```python
from build123d import *

# Parameters (mm, degrees)
F0_W     = 31.75
F0_H     = 57.15
F1_DEPTH = 50.8
F2_W     = 31.75
F2_H     = 25.4
F2_H_2   = 63.5
F3_DEPTH = 38.1
F4_W     = 63.5
F4_H     = 63.5
F5_DEPTH = 12.7
F7_DEPTH = 12.7


with BuildPart() as f1:
    # F0 (on Front) → F1 (new body)
    with BuildSketch(Plane.XZ):
        with BuildLine():
            Line((-13.088717841, 62.5215394646), (-70.238717841, 62.5215394646))
            Line((-70.238717841, 62.5215394646), (-70.238717841, 25.6915394646))
            ThreePointArc((-70.238717841, 25.6915394646), (-55.8703080473, 19.7399492583), (-49.918717841, 5.3715394646))
            Line((-49.918717841, 5.3715394646), (-13.088717841, 5.3715394646))
            Line((-13.088717841, 5.3715394646), (-13.088717841, 62.5215394646))
        make_face()
        with BuildLine():
            Line((-13.088717841, -51.7784605354), (-13.088717841, 5.3715394646))
            Line((-13.088717841, 5.3715394646), (-49.918717841, 5.3715394646))
            ThreePointArc((-49.918717841, 5.3715394646), (-55.8703080473, -8.9968703291), (-70.238717841, -14.9484605354))
            Line((-70.238717841, -14.9484605354), (-70.238717841, -51.7784605354))
            Line((-70.238717841, -51.7784605354), (-13.088717841, -51.7784605354))
        make_face()
        with BuildLine():
            Line((87.241282159, 5.3715394646), (50.411282159, 5.3715394646))
            Line((50.411282159, 5.3715394646), (50.411282159, -51.7784605354))
            Line((50.411282159, -51.7784605354), (107.561282159, -51.7784605354))
            Line((107.561282159, -51.7784605354), (107.561282159, -14.9484605354))
            ThreePointArc((107.561282159, -14.9484605354), (93.1928723653, -8.9968703291), (87.241282159, 5.3715394646))
        make_face()
        with BuildLine():
            Line((107.561282159, 62.5215394646), (50.411282159, 62.5215394646))
            Line((50.411282159, 62.5215394646), (50.411282159, 5.3715394646))
            Line((50.411282159, 5.3715394646), (87.241282159, 5.3715394646))
            ThreePointArc((87.241282159, 5.3715394646), (93.1928723653, 19.7399492583), (107.561282159, 25.6915394646))
            Line((107.561282159, 25.6915394646), (107.561282159, 62.5215394646))
        make_face()
        with Locations((2.786282159, 33.9465394646)):
            Rectangle(F0_W, F0_H)
        with Locations((2.786282159, -23.2034605354)):
            Rectangle(F0_W, F0_H)
        with Locations((34.536282159, -23.2034605354)):
            Rectangle(F0_W, F0_H)
        with Locations((34.536282159, 33.9465394646)):
            Rectangle(F0_W, F0_H)
    extrude(amount=-F1_DEPTH)

    # F2 (on face) → F3 (join)
    with BuildSketch(Plane.XZ):
        with Locations((34.536282159, 49.8215394646)):
            Rectangle(F2_W, F2_H)
        with Locations((2.786282159, 49.8215394646)):
            Rectangle(F2_W, F2_H)
        with Locations((2.786282159, -39.0784605354)):
            Rectangle(F2_W, F2_H)
        with Locations((34.536282159, -39.0784605354)):
            Rectangle(F2_W, F2_H)
        with Locations((34.536282159, 5.3715394646)):
            Rectangle(F2_W, F2_H_2)
        with Locations((2.786282159, 5.3715394646)):
            Rectangle(F2_W, F2_H_2)
    extrude(amount=F3_DEPTH)

    # F4 (on face) → F5 (cut)
    with BuildSketch(Plane.XZ.offset(38.1)):
        with Locations((18.661282159, 5.3715394646)):
            Rectangle(F4_W, F4_H)
    extrude(amount=-F5_DEPTH, mode=Mode.SUBTRACT)

    # F6 (on face) → F7 (cut)
    with BuildSketch(Plane(origin=(0, 50.8, 0), x_dir=(-1, 0, 0), z_dir=(0, 1, 0))):
        Polygon((32.138717841, 62.5215394646), (-18.661282159, 62.5215394646), (-69.461282159, 62.5215394646), (-69.461282159, -51.7784605354), (-54.4542595744, -51.7784605354), (-51.7406947911, -51.7784605354), (32.138717841, -51.7784605354), align=None)
    extrude(amount=-F7_DEPTH, mode=Mode.SUBTRACT)


solid = f1.part
```
Could you check a few things on this model? Use its own coordinates, in mm. A direction names the side the tool comes from. Give positions to 0.01 mm unless a question says otherwise; leave off trailing zeros. Write each loop counter-clockwise with the first axis right and the second up, starting at its lowest first coordinate (ties: lowest second). Pieces come first, ordered by that corner, then holes. Notation, with made-up numbers: (38, 17.25) - (76, 17.25) arc R9 cw to (76, 29.25) - close; hole circle Ø1 at (25.5, 29). An arc over 180 degrees is marked (long way). One line per item, written item: value. Start each with the question number.
Item 1: Please list where these lines run through material, in increasing order: line 1 (X direction, y = 46.5, z = 45.5); line 2 (X direction, y = -8, z = 21); line 3 (Y direction, x = -50, z = -41.5). Write a range as from..to.
Item 2: I'm going to push flat-ended pins straight in: pin 1 (10 mm diameter, centred on y = 9.5, z = 4.5, fed in from -X); pin 2 (8 mm diameter, centred on x = 85, z = -36, fed in from -Y); pin 3 (12 mm diameter, centred on y = -9, z = -37.5, fed in from -X). Where does each tip first touch, or does it pass through?
Item 3: Imagine slicing it at B-B, the plane y = 13. List the corners of the cut face in (x, z) for me.
Item 4: Imagine slicing it at C-C, the plane x = -10. List the corners of the cut face in (y, z) for me.
Item 5: Which directions (+Z, -Z, +X, -X, +Y, -Y) give clear straight access to the entire face, cutting with the end or side of a thin tool? Please do faces 1 (the face through (50.411, -15, 5)), 2 (the face through (19, 38.1, 6)), 3 (the face through (18, -32, 37.122)).
Item 6: If we mould it in two halves opening along Z, with no side actions, what happens to faces 4 (the face through (20, 16, 62.522)), 5 (the face through (-42, 0, 6)), 6 (the face through (18, -25.4, 6))? For each: +Z half, -Z half, draft (parallel to the pull), parting line (faces both ways), or undercut.
Item 7: Imagine slicing it at D-D, the plane z = -20. List the corners of the cut face in (x, y) for me.
Item 8: Imagine slicing it at A-A, the plane z = 47.5. List the corners of the cut face in (x, y) for me.
Geometry says:
1. line 1: -70.24..-32.14, 69.46..107.56
1. line 2: -13.09..50.41
1. line 3: 0..50.8
2. pin 1: x = -50.79
2. pin 2: y = 0
2. pin 3: x = -13.09
3. outline: (-70.24, -51.78) - (107.56, -51.78) - (107.56, -14.95) arc R20.32 cw to (107.56, 25.69) - (107.56, 62.52) - (-70.24, 62.52) - (-70.24, 25.69) arc R20.32 cw to (-70.24, -14.95) - close
4. outline: (-38.1, -51.78) - (38.1, -51.78) - (38.1, 62.52) - (-38.1, 62.52) - (-38.1, 37.12) - (-25.4, 37.12) - (-25.4, -26.38) - (-38.1, -26.38) - close
5. face 1: +Z, -Z, +X, -Y
5. face 2: +Z, -Z, +Y
5. face 3: +X, -X, -Y
6. face 4: +Z half
6. face 5: draft
6. face 6: undercut
7. outline: (-70.24, 0) - (-13.09, 0) - (-13.09, -25.4) - (50.41, -25.4) - (50.41, 0) - (107.56, 0) - (107.56, 50.8) - (69.46, 50.8) - (69.46, 38.1) - (-32.14, 38.1) - (-32.14, 50.8) - (-70.24, 50.8) - close
8. outline: (-70.24, 0) - (-13.09, 0) - (-13.09, -38.1) - (50.41, -38.1) - (50.41, 0) - (107.56, 0) - (107.56, 50.8) - (69.46, 50.8) - (69.46, 38.1) - (-32.14, 38.1) - (-32.14, 50.8) - (-70.24, 50.8) - close
